Source: CAD feature listing. Evaluate the final solid. Frame: model axes, mm. A direction names the side the tool comes from. Give positions to 0.01 mm unless a question says otherwise; leave off trailing zeros. Write each loop counter-clockwise with the first axis right and the second up, starting at its lowest first coordinate (ties: lowest second). Pieces come first, ordered by that corner, then holes. Notation, with made-up numbers: (-14.5, 40.5) -> (41.5, 40.5) arc R30 cw to (41.5, 70.5) -> close; hole circle Ø8 at (-33.75, 84.25). An arc over 180 degrees is marked (long way). Write item = value, one per line.
from build123d import *

# Parameters (mm, degrees)
BOSS_EXTRUDE1_DEPTH = 15.8


with BuildPart() as part:
    # Sketch1 → Boss-Extrude1 (new body)
    with BuildSketch(Plane(origin=(0, 0, 0), x_dir=(1, 0, 0), z_dir=(0, 1, 0))):
        with BuildLine():
            ThreePointArc((-3.07809394, 1.513353131), (-3.429601206, -0.052302649), (-3.030514882, -1.606511608))
            ThreePointArc((-3.030514882, -1.606511608), (-2.065248113, -2.109713097), (-1.541602156, -3.064043536))
            ThreePointArc((-1.541602156, -3.064043536), (-0.008059447, -3.429990531), (1.52718605, -3.071254266))
            ThreePointArc((1.52718605, -3.071254266), (2.055535434, -2.128465), (3.016165269, -1.633293321))
            ThreePointArc((3.016165269, -1.633293321), (3.427687897, -0.12591933), (3.127874832, 1.407586245))
            ThreePointArc((3.127874832, 1.407586245), (2.198390326, 1.972019011), (1.737882905, 2.957137637))
            ThreePointArc((1.737882905, 2.957137637), (0.056138347, 3.429540565), (-1.640166658, 3.012433125))
            ThreePointArc((-1.640166658, 3.012433125), (-2.132855627, 2.045848991), (-3.07809394, 1.513353131))
        make_face()
        Polygon((-0.9, -0.895266893), (-0.9, -2.4), (0.9, -2.4), (0.9, -0.90475813), (2.4, -0.90475813), (2.4, 0.9), (0.9, 0.9), (0.9, 2.4), (-0.9, 2.4), (-0.9, 0.9), (-2.387378381, 0.9), (-2.387378381, -0.895266893), align=None, mode=Mode.SUBTRACT)
    extrude(amount=BOSS_EXTRUDE1_DEPTH)


solid = part.part
(1) Pull-direction query (Z, two-part tool) for faces 3 (the face through (-3.43, 7.79, 0.03)), 4 (the face through (-0.9, 8, 2)), 5 (the face through (2.21, 7.79, -1.96)); classes: pulls with the +Z half, pulls with the -Z half, needs draft (parallel to the pull), parting line crosses it, or undercut.
Values follow:
face_3 = parting line crosses it
face_4 = undercut
face_5 = pulls with the -Z half
(2) Section query C-C (y = 10.25). Return loops of the section in (x, z), plus the area to 3 significant figures.
Values follow:
outline = (-3.08, -1.51) arc R1.88 cw to (-1.64, -3.01) arc R3.43 ccw to (1.74, -2.96) arc R1.88 cw to (3.13, -1.41) arc R3.43 ccw to (3.02, 1.63) arc R1.88 cw to (1.53, 3.07) arc R3.43 ccw to (-1.54, 3.06) arc R1.88 cw to (-3.03, 1.61) arc R3.43 ccw to start; hole (-2.39, -0.9) -> (-0.9, -0.9) -> (-0.9, -2.4) -> (0.9, -2.4) -> (0.9, -0.9) -> (2.4, -0.9) -> (2.4, 0.9) -> (0.9, 0.9) -> (0.9, 2.4) -> (-0.9, 2.4) -> (-0.9, 0.9) -> (-2.39, 0.9) -> close
area = 20.3 mm2
(3) Section query A-A (x = 0). Return loops of the section in (y, z).
Values follow:
outline = (0, -3.43) -> (15.8, -3.43) -> (15.8, -2.4) -> (0, -2.4) -> close; (0, 2.4) -> (15.8, 2.4) -> (15.8, 3.43) -> (0, 3.43) -> close
(4) Material intervals for line 1 (X direction, y = 9, z = 0); line 2 (Z direction, x = -2, y = 5.75); line 3 (Z direction, x = 0.75, y = 14.5), sorted ascending.
Values follow:
line_1 = -3.43 to -2.39, 2.4 to 3.43
line_2 = -2.2 to -0.9, 0.9 to 2.18
line_3 = -3.35 to -2.4, 2.4 to 3.35
(5) Section query B-B (z = -1.25). Return loops of the section in (x, y), plus the area to 3 significant figures.
Values follow:
outline = (-3.19, 0) -> (-0.9, 0) -> (-0.9, 15.8) -> (-3.19, 15.8) -> close; (0.9, 0) -> (3.19, 0) -> (3.19, 15.8) -> (0.9, 15.8) -> close
area = 72.5 mm2
(6) Access query for faces 1 (the face through (-0.03, 7.79, 3.43)), 2 (the face through (0, 8, -2.4)). Directions: +Z, -Z, +X, -X, +Y, -Y. A direction counts if a zero-diameter tool reaches every point of the face in a straight line with its end or side. Return the directions, or none.
Values follow:
face_1 = +Z, +Y, -Y
face_2 = +Y, -Y
(7) First-contact query: pin 1 (0.5 mm diameter, centred on x = 0.5, y = 8.5, fed in from -Z); pin 2 (1.2 mm diameter, centred on y = 6.5, z = 2, fed in from +X); pin 3 (1.6 mm diameter, centred on y = 9, z = 1.5, fed in from -X). Flat tips, straight axial feed; report the tip coordinate or a pass-through.
Values follow:
pin_1 = -3.42
pin_2 = 3.13
pin_3 = -3.36
(8) Section query D-D (z = -2.75). Return loops of the section in (x, y), plus the area to 3 significant figures.
Values follow:
outline = (-1.71, 0) -> (1.78, 0) -> (1.78, 15.8) -> (-1.71, 15.8) -> close
area = 55.1 mm2
